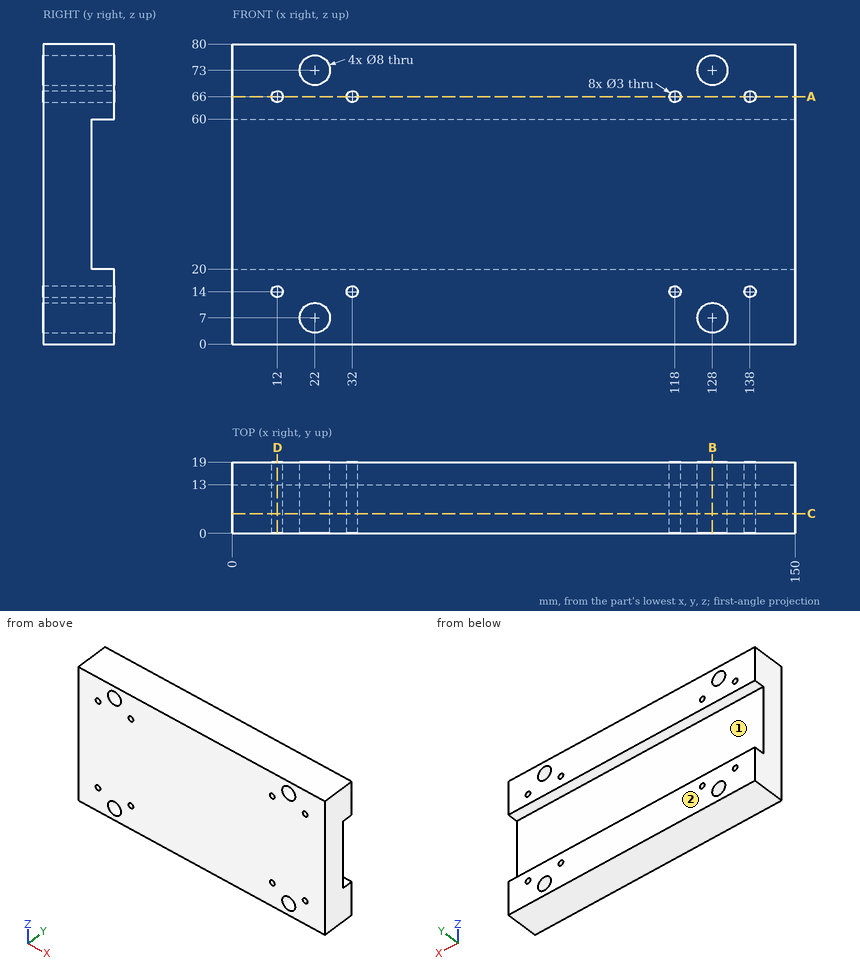
Check sheet for the drawn part. Datum: minimum x, y, z corner. Units: mm. A direction names the side the tool comes from. Give positions to 0.01 mm unless a question says otherwise; leave off trailing zeros. Loops run counter-clockwise (first coordinate to the right, second up) from the corner with the lowest first, then second, coordinate; pieces in that order, holes last.
1) Thickness scan on line 1 along Z through (x, y) = (12, 8.5); line 2 along Z through (x, y) = (107.5, 16); line 3 along Z through (x, y) = (12, 15.25). Record the ranges inside material, lowest first.
2) Sectioned sample at D-D, the plane x = 12. Enter the section's corners in (y, z).
3) Sectioned sample at B-B, the plane x = 128. Enter the section's corners in (y, z), then the cut area to 3 significant figures.
4) Sectioned sample at C-C, the plane y = 5.25. Count the separate pieces of the cut face and the enclosed holes in it, then the cut area to 3 significant figures.
5) Depth check by flat-ended pin: pin 1 Ø1.8 at (x, z) = (12, 14) entering from +Y (3 decimals); pin 2 Ø20 at (x, z) = (85.5, 33) entering from +Y. Enter the tip coordinate at first touch or a pass-through.
6) Set-up check for the marked faces 1 and 2: record each of +Z, -Z, +X, -X, +Y, -Y from which the full face is reachable in a straight line by a thin tool's end or side.
7) Sectioned sample at A-A, the plane z = 66. Enter the section's corners in (x, y).
Answers:
1. line 1: z = 0 to 12.5, 15.5 to 64.5, 67.5 to 80
1. line 2: z = 0 to 20, 60 to 80
1. line 3: z = 0 to 12.5, 15.5 to 20, 60 to 64.5, 67.5 to 80
2. outline: (0, 0) - (19, 0) - (19, 12.5) - (0, 12.5) - close; (0, 15.5) - (19, 15.5) - (19, 20) - (13, 20) - (13, 60) - (19, 60) - (19, 64.5) - (0, 64.5) - close; (0, 67.5) - (19, 67.5) - (19, 80) - (0, 80) - close
3. outline: (0, 0) - (19, 0) - (19, 3) - (0, 3) - close; (0, 11) - (19, 11) - (19, 20) - (13, 20) - (13, 60) - (19, 60) - (19, 69) - (0, 69) - close; (0, 77) - (19, 77) - (19, 80) - (0, 80) - close
3. area: 976 mm2
4. separate pieces: 1
4. enclosed holes: 12
4. area: 11,700 mm2
5. pin 1: passes through
5. pin 2: stops at y = 13
6. face 1: +X, -X, +Y
6. face 2: +Z, -Z, +X, -X, +Y
7. outline: (0, 0) - (10.5, 0) - (10.5, 19) - (0, 19) - close; (13.5, 0) - (30.5, 0) - (30.5, 19) - (13.5, 19) - close; (33.5, 0) - (116.5, 0) - (116.5, 19) - (33.5, 19) - close; (119.5, 0) - (136.5, 0) - (136.5, 19) - (119.5, 19) - close; (139.5, 0) - (150, 0) - (150, 19) - (139.5, 19) - close
